Check sheet for the modelled part. Datum: model origin and axes. Units: mm. Give positions to 0.01 mm unless a question says otherwise; leave off trailing zeros. Order: outer loops, then holes, each group sorted by start corner. A loop starts at its lowest first (then second) coordinate and runs counter-clockwise, first axis right, second up.
Item 1: Material ranges on line 1 along Z through (x, y) = (2.5, 5.25); line 2 along Z through (x, y) = (-17.5, 2.25); line 3 along X through (y, z) = (2.75, -50), recorded low to high.
Item 2: Sectioned sample at B-B on x = 52. Record the boundary of the cut face in (y, z).
Item 3: Gauge pin test, flat ends, axial feed: P1, Ø2.5, axis at x = -66, y = 1.5, coming from the -Z side; P2, Ø5.5, axis at y = 3, z = -66, coming from the +X side; P3, Ø6, axis at x = -8, y = 3.5, coming from the +Z side. Record the tip position at first contact, or that the pin passes through.
Item 4: Sectioned sample at D-D on x = -42.5. Record the boundary of the cut face in (y, z).
Item 5: Sectioned sample at C-C on z = 11. Record the boundary of the cut face in (x, y), and give its area (3 significant figures).
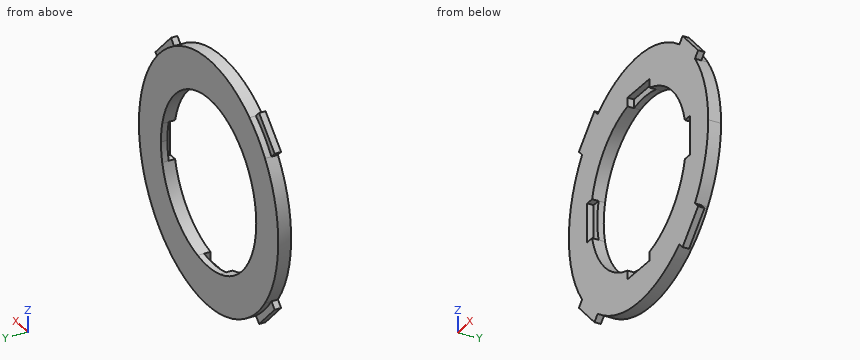
from build123d import *

# Parameters (mm, degrees)
BOSS_EXTRUDE1_DEPTH = 10
BOSS_EXTRUDE2_DEPTH = 5
BOSS_EXTRUDE3_START = 5
BOSS_EXTRUDE3_DEPTH = 5


with BuildPart() as part:
    # Sketch1 → Boss-Extrude1 (new body)
    with BuildSketch(Plane(origin=(0, 0, 0), x_dir=(1, 0, 0), z_dir=(0, 1, 0))):
        with BuildLine():
            ThreePointArc((76.939097525, 55.725894089), (67.175144213, 67.175144213), (55.725894089, 76.939097525))
            ThreePointArc((55.725894089, 76.939097525), (0, 95), (-55.725894089, 76.939097525))
            ThreePointArc((-55.725894089, 76.939097525), (-67.175144213, 67.175144213), (-76.939097525, 55.725894089))
            ThreePointArc((-76.939097525, 55.725894089), (-95, 0), (-76.939097525, -55.725894089))
            ThreePointArc((-76.939097525, -55.725894089), (-67.175144213, -67.175144213), (-55.725894089, -76.939097525))
            ThreePointArc((-55.725894089, -76.939097525), (0, -95), (55.725894089, -76.939097525))
            ThreePointArc((55.725894089, -76.939097525), (67.175144213, -67.175144213), (76.939097525, -55.725894089))
            ThreePointArc((76.939097525, -55.725894089), (90.372048402, -29.289808254), (95, 0))
            ThreePointArc((95, 0), (90.372048402, 29.289808254), (76.939097525, 55.725894089))
        make_face()
        with BuildLine():
            Line((-63.245553203, -15), (-70, -15))
            Line((-70, -15), (-70, 15))
            Line((-70, 15), (-63.245553203, 15))
            ThreePointArc((-63.245553203, 15), (-45.961940777, 45.961940777), (-15, 63.245553203))
            Line((-15, 63.245553203), (-15, 70))
            Line((-15, 70), (15, 70))
            Line((15, 70), (15, 63.245553203))
            ThreePointArc((15, 63.245553203), (45.961940777, 45.961940777), (63.245553203, 15))
            Line((63.245553203, 15), (70, 15))
            Line((70, 15), (70, -15))
            Line((70, -15), (63.245553203, -15))
            ThreePointArc((63.245553203, -15), (45.961940777, -45.961940777), (15, -63.245553203))
            Line((15, -63.245553203), (15, -70))
            Line((15, -70), (-15, -70))
            Line((-15, -70), (-15, -63.245553203))
            ThreePointArc((-15, -63.245553203), (-45.961940777, -45.961940777), (-63.245553203, -15))
        make_face(mode=Mode.SUBTRACT)
    extrude(amount=BOSS_EXTRUDE1_DEPTH)

    # Sketch1_3 → Boss-Extrude2 (add)
    with BuildSketch(Plane(origin=(0, 0, 0), x_dir=(1, 0, 0), z_dir=(0, 1, 0))):
        with BuildLine():
            ThreePointArc((-76.939097525, 55.725894089), (-67.175144213, 67.175144213), (-55.725894089, 76.939097525))
            Line((-55.725894089, 76.939097525), (-60.104076401, 81.317279836))
            Line((-60.104076401, 81.317279836), (-81.317279836, 60.104076401))
            Line((-81.317279836, 60.104076401), (-76.939097525, 55.725894089))
        make_face()
        with BuildLine():
            Line((81.317279836, 60.104076401), (60.104076401, 81.317279836))
            Line((60.104076401, 81.317279836), (55.725894089, 76.939097525))
            ThreePointArc((55.725894089, 76.939097525), (67.175144213, 67.175144213), (76.939097525, 55.725894089))
            Line((76.939097525, 55.725894089), (81.317279836, 60.104076401))
        make_face()
        with BuildLine():
            Line((81.317279836, -60.104076401), (76.939097525, -55.725894089))
            ThreePointArc((76.939097525, -55.725894089), (67.175144213, -67.175144213), (55.725894089, -76.939097525))
            Line((55.725894089, -76.939097525), (60.104076401, -81.317279836))
            Line((60.104076401, -81.317279836), (81.317279836, -60.104076401))
        make_face()
        with BuildLine():
            ThreePointArc((-55.725894089, -76.939097525), (-67.175144213, -67.175144213), (-76.939097525, -55.725894089))
            Line((-76.939097525, -55.725894089), (-81.317279836, -60.104076401))
            Line((-81.317279836, -60.104076401), (-60.104076401, -81.317279836))
            Line((-60.104076401, -81.317279836), (-55.725894089, -76.939097525))
        make_face()
    extrude(amount=BOSS_EXTRUDE2_DEPTH)

    # Sketch1_4 → Boss-Extrude3 (add)
    with BuildSketch(Plane(origin=(0, 0, 0), x_dir=(1, 0, 0), z_dir=(0, 1, 0)).offset(BOSS_EXTRUDE3_START)):
        with BuildLine():
            Line((-70, 15), (-70, -15))
            Line((-70, -15), (-63.245553203, -15))
            ThreePointArc((-63.245553203, -15), (-65, 0), (-63.245553203, 15))
            Line((-63.245553203, 15), (-70, 15))
        make_face()
        with BuildLine():
            ThreePointArc((15, -63.245553203), (0, -65), (-15, -63.245553203))
            Line((-15, -63.245553203), (-15, -70))
            Line((-15, -70), (15, -70))
            Line((15, -70), (15, -63.245553203))
        make_face()
        with BuildLine():
            Line((-15, 70), (-15, 63.245553203))
            ThreePointArc((-15, 63.245553203), (0, 65), (15, 63.245553203))
            Line((15, 63.245553203), (15, 70))
            Line((15, 70), (-15, 70))
        make_face()
        with BuildLine():
            ThreePointArc((65, 0), (64.559898382, -7.551127127), (63.245553203, -15))
            Line((63.245553203, -15), (70, -15))
            Line((70, -15), (70, 15))
            Line((70, 15), (63.245553203, 15))
            ThreePointArc((63.245553203, 15), (64.559898382, 7.551127127), (65, 0))
        make_face()
    extrude(amount=BOSS_EXTRUDE3_DEPTH)


solid = part.part
Report:
1. line 1: z = -94.97 to -64.95, 64.95 to 94.97
1. line 2: z = -93.37 to -62.6, 62.6 to 93.37
1. line 3: x = -80.78 to -41.53, 41.53 to 80.78
2. outline: (0, -79.5) - (10, -79.5) - (10, -39) - (0, -39) - close; (0, 39) - (10, 39) - (10, 79.5) - (0, 79.5) - close
3. P1: stops at z = -76.67
3. P2: stops at x = 78.17
3. P3: stops at z = 94.87
4. outline: (0, -84.96) - (10, -84.96) - (10, -49.18) - (0, -49.18) - close; (0, 49.18) - (10, 49.18) - (10, 84.96) - (0, 84.96) - close
5. outline: (-94.36, 0) - (-70, 0) - (-70, 5) - (-64.06, 5) - (-64.06, 10) - (-94.36, 10) - close; (64.06, 5) - (70, 5) - (70, 0) - (94.36, 0) - (94.36, 10) - (64.06, 10) - close
5. area: 547 mm2
